Autodesk Inventor part; units mm, degrees
ref_plane "YZ Plane" through (0, 0, 0) normal (1, 0, 0) x (0, 1, 0)
ref_plane "XZ Plane" through (0, 0, 0) normal (0, 1, 0) x (-1, 0, 0)
ref_plane "XY Plane" through (0, 0, 0) normal (0, 0, 1) x (1, 0, 0)
sketch "Sketch1" plane through (0, 0, 0) normal (0, 0, 1) x (1, 0, 0)
  circle A0 centre (0, 0) radius 6.35
  dimension "d0" = 12.7
extrude "Extrusion1" add sketch "Sketch1" along normal mid plane 152.4
sketch "Sketch2" plane through (0, 0, 76.2) normal (0, 0, 1) x (1, 0, 0)
  circle A0 centre (0, 0) radius 6.35
  circle A1 centre (0, 0) radius 3.175
  dimension "d3" = 6.35
extrude "Extrusion2" cut sketch "Sketch2" against normal blind 139.7 contours A1
fillet "Fillet1" radius 3.175 2 edges at (-6.35, 0, -76.2) (-6.35, 0, 76.2)
sketch "Sketch3" plane through (0, 0, -76.2) normal (0, 0, -1) x (-1, 0, 0)
  circle A0 centre (0, 0) radius 3.175
  line L0 (-1.1906, 2.9433) -> (-1.1906, -2.9433)
  line L1 (1.1906, 2.9433) -> (1.1906, -2.9433)
  line L2 (0, -8.89) -> (0, 8.89)
  line L3 (-1.1906, 2.9433) -> (1.1906, 2.9433)
  line L4 (1.1906, -2.9433) -> (-1.1906, -2.9433)
  dimension "d7" = 2.3813
extrude "Extrusion3" add sketch "Sketch3" along normal blind 6.35 contours L1 L4 L2 L3 | L2 L4 L0 L3
sketch "Sketch4" plane through (-1.1906, -2.9433, -76.2) normal (-1, 0, 0) x (0, 0, 1)
  line L0 (-6.35, 5.8866) -> (-6.35, 0)
  line L1 (0, 0) -> (-6.35, 0)
  line L2 (0, 5.8866) -> (0, 0)
  line L3 (0, 5.8866) -> (-6.35, 5.8866)
  arc A0 (-3.4067, 5.8866) -> (-3.4067, 0) centre (-3.4067, 2.9433) ccw
  point P0 (76.2, 2.9433)
extrude "Extrusion4" cut sketch "Sketch4" against normal through all contours L3 A0 L0 | A0 L1 L0
properties part number "piston_outer"
The listing builds one solid part. Answer for the finished solid, in the listing's coordinates (mm). A direction names the side the tool comes from. Coordinates: 2 decimals unless noted, no trailing zeros. Loops run counter-clockwise (first coordinate to the right, second up) from the corner with the lowest first, then second, coordinate; pieces in that order, holes last. Notation, with made-up numbers: (-16.75, -33) - (38.25, -33) arc R33 ccw to (38.25, -2) - close; hole circle Ø3 at (-10, 75). An arc over 180 degrees is marked (long way). Use a Markdown table: item, result. Add a question column.
1) The part is cut by section B-B, the plane z = 22. Give the vertices of the cut face in (x, y) (3 decimals), and give its area (3 significant figures).
2) The mould has two halves that part along X. Classify faces 4 (the cylindrical face through (-0.69, -3.1, 7.33)), 5 (the cylindrical face through (-1.38, -6.2, 1.02)), 6 (the flat face through (1.191, 0, -79)): released by +X, released by -X, zero draft, split by the parting line, or undercut.
3) Given pin 1 (4 mm diameter, centred on x = 5, y = 3, fed in from -Z); pin 2 (7 mm diameter, centred on x = 0, y = -1, fed in from -Z); pin 3 (3 mm diameter, centred on y = -5, z = -2, fed in from +X); pin 4 (3 mm diameter, centred on x = 0.5, y = -1.5, fed in from +Z), each flat-ended and moving along its own axis, determine where each tip first touches the part or whether it passes through.
4) Find the intervals of material crossed by line 1 (Y direction, x = 0, z = -3.5) (3 decimals); line 2 (Z direction, x = 1.75, y = -2.75); line 3 (Y direction, x = 2.25, z = 30), in increasing order.
5) For faces 1 (the cylindrical face through (-0.02, 0.06, -82.55)), 2 (the flat face through (-1.191, 0, -79)), 3 (the flat face through (0, 0, -63.5)), determine the directions among +Z, -Z, +X, -X, +Y, -Y from which every point of the face is accessible in a straight line to the end or side of a thin tool.
Here are the results:
| question | item | result |
|---|---|---|
| 1 | outline | circle Ø12.7 at (0, 0); hole circle Ø6.35 at (0, 0) |
| 1 | area | 95.0 mm^2 |
| 2 | face 4 | undercut |
| 2 | face 5 | split by the parting line |
| 2 | face 6 | released by +X |
| 3 | pin 1 | stops at z = -76.13 |
| 3 | pin 2 | stops at z = -82.55 |
| 3 | pin 3 | stops at x = 5.3 |
| 3 | pin 4 | stops at z = -63.5 |
| 4 | line 1 | y = -6.35 to -3.175, 3.175 to 6.35 |
| 4 | line 2 | z = -76.2 to 76.2 |
| 4 | line 3 | y = -5.94 to -2.24, 2.24 to 5.94 |
| 5 | face 1 | -Z, +X, -X |
| 5 | face 2 | -Z, -X, +Y, -Y |
| 5 | face 3 | +Z |
